Check sheet for the drawn part. Datum: minimum x, y, z corner. Units: mm. Give positions to 0.01 mm unless a question says otherwise; leave off trailing zeros. Write each loop counter-clockwise with the first axis right and the second up, starting at its lowest first coordinate (ties: lowest second). Pieces come first, ordered by that corner, then holes. Notation, with made-up numbers: M -3.5,61 L 48.5,61 A11 ccw 48.5,70 Z; hole C -14,73 d7. An arc over 180 degrees is marked long. Write item = value, one per line. Start each with the question number.
1) Scan lines: L1, parallel to X at y = 9, z = 65; L2, parallel to Y at x = 20, z = 37; L3, parallel to Y at x = 41, z = 24.5. Record each from-to range of solid material in increasing order.
2) Gauge pin test, flat ends, axial feed: pin 1 (21 mm diameter, centred on y = 11, z = 30, fed in from -X); pin 2 (10 mm diameter, centred on y = 42, z = 73, fed in from -X); pin 3 (5 mm diameter, centred on x = 6.5, z = 52.5, fed in from +Y); pin 4 (12 mm diameter, centred on x = 44, y = 13.5, fed in from -Z). Record the tip position at first contact, or that the pin passes through.
3) Sectioned sample at C-C, the plane z = 69. Record the cut outline in (x, y).
4) Sectioned sample at A-A, the plane x = 26. Record the cut outline in (y, z), then the cut area to 3 significant figures.
5) Draft check along X on the marked faces 1 and 2. Enter one of: pulls with the +X half, pulls with the -X half, needs draft (parallel to the pull), parting line crosses it, or undercut.
6) Sectioned sample at D-D, the plane x = 16.5. Record the cut outline in (y, z).
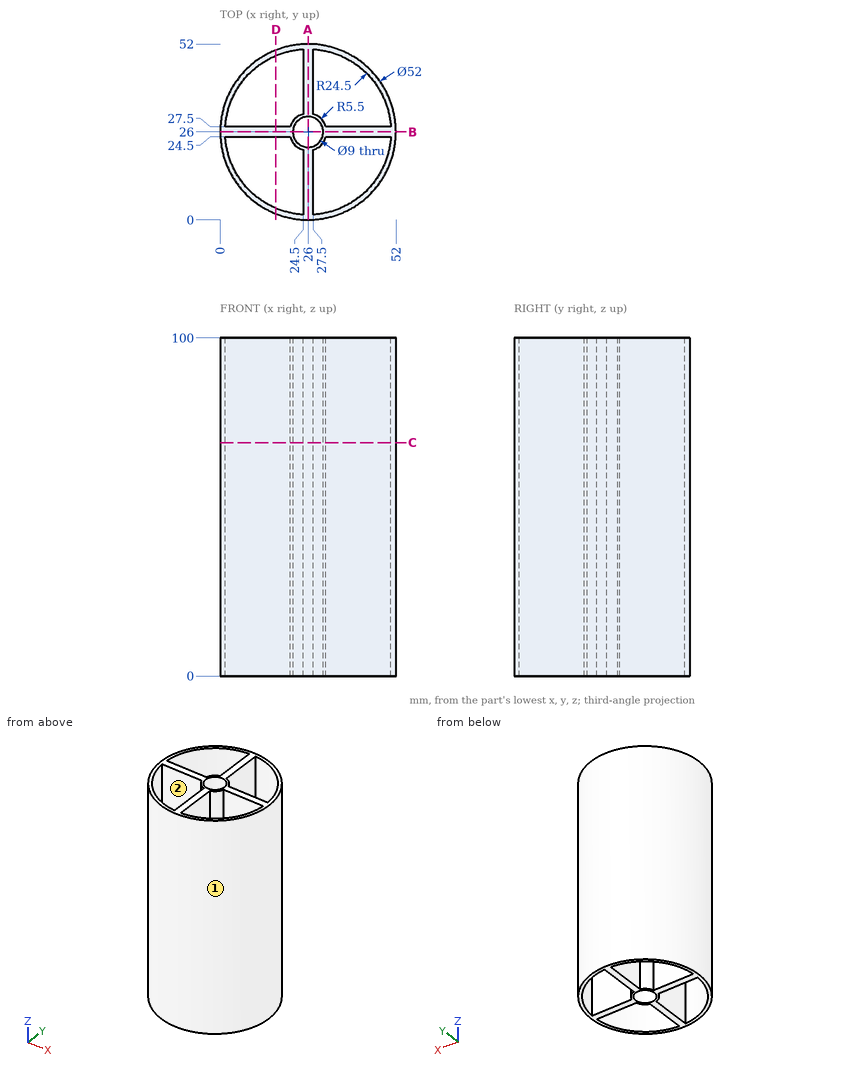
Data:
q1.L1 = 6.33 to 8.36, 24.5 to 27.5, 43.64 to 45.67
q1.L2 = 0.7 to 2.25, 24.5 to 27.5, 49.75 to 51.3
q1.L3 = 4.76 to 6.63, 24.5 to 27.5, 45.37 to 47.24
q2.pin_1 = 0.39
q2.pin_2 = 2.44
q2.pin_3 = 45.67
q2.pin_4 = 0
q3.outline = C 26,26 d52; hole M 1.55,24.5 A24.5 ccw 24.5,1.55 L 24.5,20.71 A5.5 cw 20.71,24.5 Z; hole M 1.55,27.5 L 20.71,27.5 A5.5 cw 24.5,31.29 L 24.5,50.45 A24.5 ccw Z; hole C 26,26 d9; hole M 27.5,1.55 A24.5 ccw 50.45,24.5 L 31.29,24.5 A5.5 cw 27.5,20.71 Z; hole M 27.5,31.29 A5.5 cw 31.29,27.5 L 50.45,27.5 A24.5 ccw 27.5,50.45 Z
q4.outline = M 0,0 L 21.5,0 L 21.5,100 L 0,100 Z; M 30.5,0 L 52,0 L 52,100 L 30.5,100 Z
q4.area = 4,300 mm2
q5.face_1 = parting line crosses it
q5.face_2 = undercut
q6.outline = M 1.8,0 L 3.42,0 L 3.42,100 L 1.8,100 Z; M 24.5,0 L 27.5,0 L 27.5,100 L 24.5,100 Z; M 48.58,0 L 50.2,0 L 50.2,100 L 48.58,100 Z
